```python
from build123d import *

# Parameters (mm, degrees)
BOSS_EXTRUDE1_DEPTH = 2.2
SKETCH2_W           = 1
SKETCH2_H           = 0.2
SKETCH4_W           = 2.6
SKETCH4_H           = 0.2
SKETCH6_R           = 0.5
BOSS_EXTRUDE2_DEPTH = 1.2


with BuildPart() as part:
    # Sketch1 → Boss-Extrude1 (new body)
    with BuildSketch(Plane.XY):
        with BuildLine():
            Line((0, 5.3), (2.6, 5.3))
            Line((2.6, 5.3), (4.2, 3.35))
            Line((4.2, 3.35), (4.2, 2.35))
            Line((4.2, 2.35), (5.3, 2.35))
            Line((5.3, 2.35), (5.3, -2.35))
            Line((5.3, -2.35), (4.2, -2.35))
            Line((4.2, -2.35), (4.2, -7.35))
            Line((4.2, -7.35), (0, -7.35))
            Line((0, -7.35), (0, -2.5))
            ThreePointArc((0, -2.5), (2.5, 0), (0, 2.5))
            Line((0, 2.5), (0, 5.3))
        make_face()
    boss_extrude1 = extrude(amount=BOSS_EXTRUDE1_DEPTH)

    # Mirror1: Boss-Extrude1 across plane
    add(boss_extrude1.mirror(Plane(origin=(0, -7.35, 2.2), x_dir=(0, 0, 1), z_dir=(1, 0, 0))))

    # Sweep1: sweep along a path in Sketch3
    with BuildLine(Plane(origin=(0, 0, 0), x_dir=(0, 0, -1), z_dir=(1, 0, 0))) as sweep1_path:
        Line((-2, -7.35), (-2, -7.549456001))
        ThreePointArc((-2, -7.549456001), (-1.908338682, -7.770745997), (-1.687048686, -7.862407315))
        Line((-1.687048686, -7.862407315), (-0.312951314, -7.862407315))
        ThreePointArc((-0.312951314, -7.862407315), (-0.091661318, -7.954068633), (0, -8.17535863))
        Line((0, -8.17535863), (0, -8.725))
    # Sketch2 → Sweep1 (sweep)
    with BuildSketch(Plane.XZ.offset(7.35)):
        with Locations((-2.5, 2.1)):
            Rectangle(SKETCH2_W, SKETCH2_H)
        with Locations((0, 2.1)):
            Rectangle(SKETCH2_W, SKETCH2_H)
        with Locations((2.5, 2.1)):
            Rectangle(SKETCH2_W, SKETCH2_H)
    sweep(path=sweep1_path.line)

    # Sweep2: sweep along a path in Sketch5
    with BuildLine(Plane(origin=(0, 0, 0), x_dir=(0, 0, -1), z_dir=(1, 0, 0))) as sweep2_path:
        Line((-2.060981918, 5.3), (-2.060981918, 5.452016603))
        ThreePointArc((-2.060981918, 5.452016603), (-2.002498709, 5.59320756), (-1.861307752, 5.651690769))
        Line((-1.861307752, 5.651690769), (-0.199674166, 5.651690769))
        ThreePointArc((-0.199674166, 5.651690769), (-0.058483209, 5.710173978), (0, 5.851364935))
        Line((0, 5.851364935), (0, 6.675))
    # Sketch4 → Sweep2 (sweep)
    with BuildSketch(Plane(origin=(0, 5.3, 0), x_dir=(1, 0, 0), z_dir=(0, 1, 0))):
        with Locations((0, -2.1)):
            Rectangle(SKETCH4_W, SKETCH4_H)
    sweep(path=sweep2_path.line)

    # Sketch6 → Boss-Extrude2 (add)
    with BuildSketch(Plane(origin=(0, 0, 0), x_dir=(-1, 0, 0), z_dir=(0, 0, -1))):
        with Locations((-4.2, 0)):
            Circle(SKETCH6_R)
        with Locations((4.2, 0)):
            Circle(SKETCH6_R)
    extrude(amount=BOSS_EXTRUDE2_DEPTH)


solid = part.part
```
Check sheet for the modelled part. Datum: model origin and axes. Units: mm. A direction names the side the tool comes from. Give positions to 0.01 mm unless a question says otherwise; leave off trailing zeros. Order: outer loops, then holes, each group sorted by start corner. A loop starts at its lowest first (then second) coordinate and runs counter-clockwise, first axis right, second up. Notation, with made-up numbers: (-11.75, 51) -> (-2.75, 51) arc R25 cw to (-2.75, 79) -> close; hole circle Ø5 at (54, 33.5). An arc over 180 degrees is marked (long way). Use CSV: the item, a comma, the result in double quotes. Start each with the question number.
1) Set-up check for faces 5 (the face through (0, 5.791, 1)), 6 (the face through (0, 5.591, 1)), 7 (the face through (3.723, 0.15, -0.592)): record each of +Z, -Z, +X, -X, +Y, -Y from which the full face is reachable in a straight line by a thin tool's end or side.
2) Sectioned sample at C-C, the plane y = 3. Record the boundary of the cut face in (x, z).
3) Go/stop test with flat-tipped pins: P1, Ø0.5, axis at x = 0, z = 1, coming from the +Y side; P2, Ø1.8, axis at y = -4.5, z = 1.5, coming from the -X side; P3, Ø1.2, axis at x = 5, z = 1.5, coming from the +Y side. Record where each tip stops, or that it passes through.
4) Mould release check, pull along Y, two halves, no side actions. Record for faces 1 (the face through (2.5, -7.862, 1)), 2 (the face through (-2.5, -8.062, 1)), 3 (the face through (-4.2, 3, 1)), 4 (the face through (-2.5, -7.862, 1)): released by +Y, released by -Y, zero draft, split by the parting line, or undercut.
5) Sectioned sample at A-A, the plane z = 0.5. Give the number of separate pieces and of enclosed holes in the cut face, plus the area to 3 significant figures.
6) Material ranges on line 1 (Y direction, x = -1.5, z = 1.65); line 2 (Y direction, x = -0.75, z = 1.4); line 3 (Y direction, x = -2.25, z = 1.4), recorded low to high. Write a range as from..to.
7) Sectioned sample at B-B, the plane y = 0. Record the boundary of the cut face in (x, z), plus the area to 3 significant figures.
Recorded:
1,face 5,"+Z, +X, -X, +Y"
1,face 6,"-Z, +X, -X"
1,face 7,"-Z"
2,outline,"(-4.2, 0) -> (4.2, 0) -> (4.2, 2.2) -> (-4.2, 2.2) -> close"
3,P1,"y = 5.79"
3,P2,"x = -4.2"
3,P3,"y = 2.35"
4,face 1,"undercut"
4,face 2,"released by -Y"
4,face 3,"zero draft"
4,face 4,"undercut"
5,separate pieces,"5"
5,enclosed holes,"1"
5,area,"95.0 mm2"
6,line 1,"-7.35..-2, 2..5.3"
6,line 2,"-7.35..-2.38, 2.38..5.3, 5.59..5.79"
6,line 3,"-8.06..-7.86, -7.35..-1.09, 1.09..5.3"
7,outline,"(-5.3, 0) -> (-4.7, 0) -> (-4.7, -1.2) -> (-3.7, -1.2) -> (-3.7, 0) -> (-2.5, 0) -> (-2.5, 2.2) -> (-5.3, 2.2) -> close; (2.5, 0) -> (3.7, 0) -> (3.7, -1.2) -> (4.7, -1.2) -> (4.7, 0) -> (5.3, 0) -> (5.3, 2.2) -> (2.5, 2.2) -> close"
7,area,"14.7 mm2"
